Design review of the part built by this model. Coordinates are the model's own, in mm. Face numbers are marked on the shaded views. A direction names the side the tool comes from. Coordinates: 2 decimals unless noted, no trailing zeros. Order: outer loops, then holes, each group sorted by start corner. A loop starts at its lowest first (then second) coordinate and runs counter-clockwise, first axis right, second up.
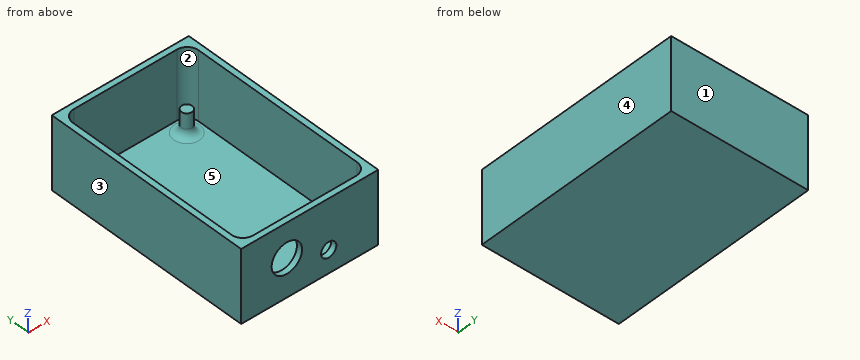
from build123d import *

# Parameters (mm, degrees)
SKETCH_W        = 36
SKETCH_H        = 55
PAD_DEPTH       = 19
SKETCH001_W     = 33
SKETCH001_H     = 52
POCKET_DEPTH    = 18
SKETCH002_R     = 1.4
PAD001_DEPTH    = 6
SKETCH003_R     = 4
SKETCH003_R_2   = 2
POCKET001_DEPTH = 1.5
FILLET_R        = 2
FILLET001_R     = 3


with BuildPart() as part:
    # Sketch → Pad (new body)
    with BuildSketch(Plane.XY):
        Rectangle(SKETCH_W, SKETCH_H)
    extrude(amount=PAD_DEPTH)

    # Sketch001 (on Face6 of Pad) → Pocket (cut)
    with BuildSketch(Plane.XY.offset(19)):
        Rectangle(SKETCH001_W, SKETCH001_H)
    extrude(amount=-POCKET_DEPTH, mode=Mode.SUBTRACT)

    # Sketch002 (on Face11 of Pocket) → Pad001 (join)
    with BuildSketch(Plane.XY.offset(1)):
        with Locations((-12.5, 22)):
            Circle(SKETCH002_R)
    pad001 = extrude(amount=PAD001_DEPTH)

    # Mirrored: Pad001 across Sketch002 V_Axis
    add(pad001.mirror(Plane(origin=(0, 0, 1), x_dir=(0, 0, 1), z_dir=(1, 0, 0))))

    # Sketch003 (on Face6 of Mirrored) → Pocket001 (cut)
    with BuildSketch(Plane.XZ.offset(27.5)):
        with Locations((-6, 10)):
            Circle(SKETCH003_R)
        with Locations((5, 6)):
            Circle(SKETCH003_R_2)
    extrude(amount=-POCKET001_DEPTH, mode=Mode.SUBTRACT)

    # Fillet
    fillet_edges = [part.edges().sort_by_distance(p)[0] for p in [
        (-13.9, 22, 1),
        (13.9, 22, 1),
    ]]
    fillet(fillet_edges, radius=FILLET_R)

    # Fillet001
    fillet001_edges = [part.edges().sort_by_distance(p)[0] for p in [
        (-16.5, 26, 10),
        (-16.5, -26, 10),
        (16.5, -26, 10),
        (16.5, 26, 10),
    ]]
    fillet(fillet001_edges, radius=FILLET001_R)


solid = part.part
1. Mouldability with a two-part tool opening along X and no side actions: class the marked faces 1, 2 and 3 as pulls with the +X half, pulls with the -X half, needs draft (parallel to the pull), parting line crosses it, or undercut.
2. For the marked faces 4 and 5, list the 3-axis set-ups (+Z, -Z, +X, -X, +Y, -Y) from which the entire face can be reached by the end or side of a thin tool; tool diameter is ignored.
3. Add section D-D (x = 12.5). Give the boundary of the cut face in (y, z).
4. Add section C-C (z = 12.25). Give the boundary of the cut face in (x, y), and give its area (3 significant figures).
5. To check wall thickness, follow line 1 (Y direction, x = -1, z = 13.5); line 2 (Y direction, x = 12, z = 6.5); line 3 (X direction, y = -19, z = 11.75). State the ranges of each line that lie inside material, in increasing order.
6. Add section A-A (x = 5). Give the boundary of the cut face in (y, z), and give its area (3 significant figures).
7. Add section B-B (y = 22). Give the boundary of the cut face in (x, z), and give its area (3 significant figures).
8. Insertion check: pin 1 (1.4 mm diameter, centred on x = 13, y = 22.5, fed in from +Z); pin 2 (6 mm diameter, centred on x = -2, y = -16, fed in from +Z). Each pin has a flat end and moves straight along its axis. Give the tip position at first contact, or say it passes through.
Solution:
1. face 1: needs draft
1. face 2: undercut
1. face 3: pulls with the -X half
2. face 4: +Z, -Z, +X, +Y, -Y
2. face 5: +Z
3. outline: (-27.5, 0) - (27.5, 0) - (27.5, 19) - (26, 19) - (26, 1) - (25.4, 1) arc R2 cw to (23.4, 3) - (23.4, 7) - (20.6, 7) - (20.6, 3) arc R2 cw to (18.6, 1) - (-26, 1) - (-26, 19) - (-27.5, 19) - close
4. outline: (-18, -27.5) - (-9.31, -27.5) - (-9.31, -26) - (-13.5, -26) arc R3 cw to (-16.5, -23) - (-16.5, 23) arc R3 cw to (-13.5, 26) - (13.5, 26) arc R3 cw to (16.5, 23) - (16.5, -23) arc R3 cw to (13.5, -26) - (-2.69, -26) - (-2.69, -27.5) - (18, -27.5) - (18, 27.5) - (-18, 27.5) - close
4. area: 262 mm2
5. line 1: y = -27.5 to -26, 26 to 27.5
5. line 2: y = -27.5 to -26, 20.69 to 23.31, 26 to 27.5
5. line 3: x = -18 to -16.5, 16.5 to 18
6. outline: (-27.5, 0) - (27.5, 0) - (27.5, 19) - (26, 19) - (26, 1) - (-26, 1) - (-26, 4) - (-27.5, 4) - close; (-27.5, 8) - (-26, 8) - (-26, 19) - (-27.5, 19) - close
6. area: 103 mm2
7. outline: (-18, 0) - (18, 0) - (18, 19) - (16.5, 19) - (16.5, 1) - (15.9, 1) arc R2 cw to (13.9, 3) - (13.9, 7) - (11.1, 7) - (11.1, 3) arc R2 cw to (9.1, 1) - (-9.1, 1) arc R2 cw to (-11.1, 3) - (-11.1, 7) - (-13.9, 7) - (-13.9, 3) arc R2 cw to (-15.9, 1) - (-16.5, 1) - (-16.5, 19) - (-18, 19) - close
7. area: 127 mm2
8. pin 1: stops at z = 7
8. pin 2: stops at z = 1
